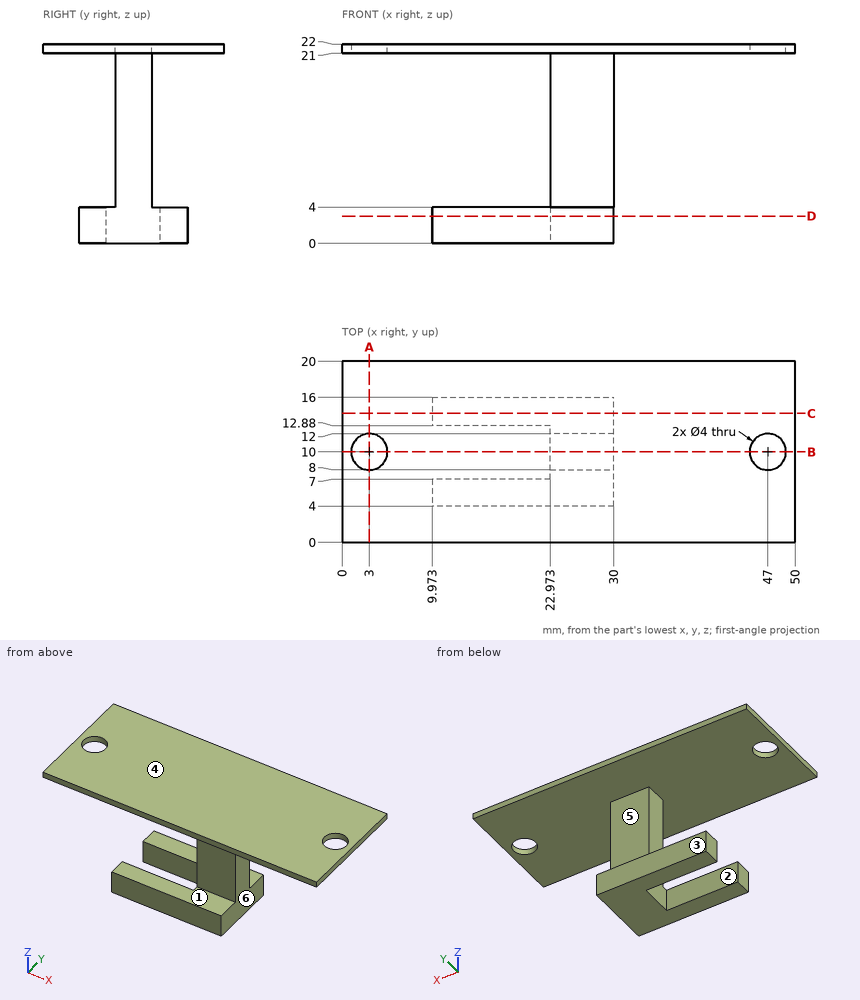
Design review of the part shown in the three views and the two pictorial views. Dimensions are in mm from the part's minimum x, y and z. A direction names the side the tool comes from. Give positions to 0.01 mm unless a question says otherwise; leave off trailing zeros. Loops run counter-clockwise (first coordinate to the right, second up) from the corner with the lowest first, then second, coordinate; pieces in that order, holes last. Notation, with made-up numbers: (67, -4.5) -> (119, -4.5) arc R16 cw to (119, 3.5) -> close; hole circle Ø3 at (70, 76.25). An arc over 180 degrees is marked (long way). Put each result on its own line as item: value. Start each with the question number.
1. We need section A-A on x = 3. State the section outline as (y, z) points.
2. We need section B-B on y = 10. State the section outline as (x, z) points.
3. For the marked faces 1, 2 and 3, list the 3-axis set-ups (+Z, -Z, +X, -X, +Y, -Y) from which the entire face can be reached by the end or side of a thin tool; tool diameter is ignored.
4. Wall thickness on probe 1 along X at (y, z) = (10, 21.45); probe 2 along Y at (x, z) = (47, 21.25); probe 3 along Z at (x, y) = (48, 6.5): over which ranges is each line inside the solid? List them lowest first.
5. We need section C-C on y = 14.25. State the section outline as (x, z) points.
6. We need section D-D on z = 3. State the section outline as (x, y) points.
7. Clearance check with flat-ended pins moving along their axes: P1, Ø3.5, axis at y = 14.5, z = 1.5, coming from the -X side; P2, Ø1.2, axis at x = 16.5, z = 2, coming from the +Y side; P3, Ø8, axis at x = 40.5, z = 15.5, coming from the +Y side; P4, Ø3, axis at x = 19, z = 1.5, coming from the -Y side. State where each tip first meets the part, or that it passes through.
8. Mouldability with a two-part tool opening along Z and no side actions: class the marked faces 4, 5 and 6 as released by +Z, released by -Z, zero draft, split by the parting line, or undercut.
Determined:
1. outline: (0, 21) -> (8, 21) -> (8, 22) -> (0, 22) -> close; (12, 21) -> (20, 21) -> (20, 22) -> (12, 22) -> close
2. outline: (0, 21) -> (1, 21) -> (1, 22) -> (0, 22) -> close; (5, 21) -> (22.97, 21) -> (22.97, 0) -> (30, 0) -> (30, 21) -> (45, 21) -> (45, 22) -> (5, 22) -> close; (49, 21) -> (50, 21) -> (50, 22) -> (49, 22) -> close
3. face 1: +X, -X, -Y
3. face 2: -Z, -X
3. face 3: -Z, +X, -X, +Y
4. probe 1: 0 to 1, 5 to 45, 49 to 50
4. probe 2: 0 to 8, 12 to 20
4. probe 3: 21 to 22
5. outline: (0, 21) -> (50, 21) -> (50, 22) -> (0, 22) -> close; (9.97, 0) -> (30, 0) -> (30, 4) -> (9.97, 4) -> close
6. outline: (9.97, 4) -> (30, 4) -> (30, 16) -> (9.97, 16) -> (9.97, 12.88) -> (22.97, 12.88) -> (22.97, 7) -> (9.97, 7) -> close
7. P1: x = 9.97
7. P2: y = 16
7. P3: through
7. P4: y = 4
8. face 4: released by +Z
8. face 5: undercut
8. face 6: zero draft
